```python
from build123d import *

# Parameters (mm, degrees)
BOSS_EXTRU_1_DEPTH      = 3
ESQUISSE2_R             = 2
ENL_V_MAT_EXTRU_1_DEPTH = 179.997905016
CHANFREIN1_SIZE         = 40


with BuildPart() as part:
    # Esquisse1 → Boss.-Extru.1 (new body)
    with BuildSketch(Plane.XY):
        Polygon((-40, 117.5), (-40, 44.5), (40, 44.5), (40, 117.5), (135, 117.5), (135, -117.5), (40, -117.5), (40, -44.5), (-40, -44.5), (-40, -117.5), (-135, -117.5), (-135, 117.5), align=None)
    extrude(amount=BOSS_EXTRU_1_DEPTH)

    # Esquisse2 → Enlèv. mat.-Extru.1 (cut, through all)
    with BuildSketch(Plane.XY.offset(3)):
        with Locations((-17.5, -35.98)):
            Circle(ESQUISSE2_R)
        with Locations((17.5, -35.98)):
            Circle(ESQUISSE2_R)
        with Locations((-17.5, -7.98)):
            Circle(ESQUISSE2_R)
        with Locations((-17.5, 7.5)):
            Circle(ESQUISSE2_R)
        with Locations((17.5, 7.5)):
            Circle(ESQUISSE2_R)
        with Locations((17.5, -7.98)):
            Circle(ESQUISSE2_R)
        with Locations((-17.5, 35.5)):
            Circle(ESQUISSE2_R)
        with Locations((17.5, 35.5)):
            Circle(ESQUISSE2_R)
    extrude(amount=-ENL_V_MAT_EXTRU_1_DEPTH, mode=Mode.SUBTRACT)

    # Chanfrein1
    chanfrein1_edges = [part.edges().sort_by_distance(p)[0] for p in [
        (135, -117.5, 1.5),
        (-135, -117.5, 1.5),
    ]]
    chamfer(chanfrein1_edges, length=CHANFREIN1_SIZE)


solid = part.part
```
The model under review builds one solid part; all positions refer to its coordinate system, in mm. Give positions to 0.01 mm unless a question says otherwise; leave off trailing zeros. Write each loop counter-clockwise with the first axis right and the second up, starting at its lowest first coordinate (ties: lowest second). Pieces come first, ordered by that corner, then holes.
(1) To check wall thickness, follow L1, parallel to Y at x = 17.5, z = 1.75; L2, parallel to X at y = -58, z = 2.65; L3, parallel to X at y = -8.5, z = 2.8. State the ranges of each line that lie inside material, in increasing order.
(2) Consider section C-C, the plane x = 1. Give the boundary of the cut face in (y, z).
(3) Consider section B-B, the plane z = 1.85. Give the number of separate pieces and of enclosed holes in the cut face, and give its area (3 significant figures).
(4) Consider section A-A, the plane y = 92.5. Give the boundary of the cut face in (x, z).
(5) For P1, Ø1.5, axis at x = -11, z = 1.5, coming from the +Y side; P2, Ø0.9, axis at y = -83.5, z = 1.5, coming from the -X side, all flat-tipped, find the tip position at first contact; note any pin that passes through.
Returned:
1. L1: y = -44.5 to -37.98, -33.98 to -9.98, -5.98 to 5.5, 9.5 to 33.5, 37.5 to 44.5
1. L2: x = -135 to -40, 40 to 135
1. L3: x = -135 to -19.43, -15.57 to 15.57, 19.43 to 135
2. outline: (-44.5, 0) - (44.5, 0) - (44.5, 3) - (-44.5, 3) - close
3. separate pieces: 1
3. enclosed holes: 8
3. area: 50,100 mm2
4. outline: (-135, 0) - (-40, 0) - (-40, 3) - (-135, 3) - close; (40, 0) - (135, 0) - (135, 3) - (40, 3) - close
5. P1: stops at y = 44.5
5. P2: stops at x = -129.45
